```python
from build123d import *

# Parameters (mm, degrees)
F0_W     = 23.65
F0_H     = 51.55
F1_DEPTH = 35
F3_DEPTH = 23.651
F5_DEPTH = 6.25
F6_W     = 16.5
F6_H     = 4.038704
F7_DEPTH = 6.25


with BuildPart() as f1:
    # F0 (on Top) → F1 (new body)
    with BuildSketch(Plane.XY):
        with Locations((0.764201, -25.775)):
            Rectangle(F0_W, F0_H)
    extrude(amount=F1_DEPTH)

    # F2 (on face) → F3 (cut, through all)
    with BuildSketch(Plane.YZ.offset(12.589201)):
        Polygon((0, 28.75), (0, 35), (-15.663622, 35), (-11.5, 28.75), align=None)
    extrude(amount=-F3_DEPTH, mode=Mode.SUBTRACT)

    # F4 (on face) → F5 (cut)
    with BuildSketch(Plane.XY.offset(35)):
        Polygon((-4.985799, -47.763622), (0.764201, -47.763622), (6.514201, -47.763622), (9.014201, -43.008048), (9.014201, -15.663622), (0.764201, -15.663622), (-7.485799, -15.663622), (-7.485799, -43.008048), align=None)
    extrude(amount=-F5_DEPTH, mode=Mode.SUBTRACT)

    # F6 (on face) → F7 (cut)
    with BuildSketch(Plane.XY.offset(35)):
        with Locations((0.764201, -13.64427)):
            Rectangle(F6_W, F6_H)
    extrude(amount=-F7_DEPTH, mode=Mode.SUBTRACT)


solid = f1.part
```
Work out the finished part from the listing and answer in its coordinate system (mm). A direction names the side the tool comes from. Coordinates: 2 decimals unless noted, no trailing zeros. Loops run counter-clockwise (first coordinate to the right, second up) from the corner with the lowest first, then second, coordinate; pieces in that order, holes last. Notation, with made-up numbers: (70, -7) - (118, -7) arc R17 ccw to (118, 11) - close; hole circle Ø11 at (-16, 30). An arc over 180 degrees is marked (long way). Use a Markdown table: item, result.
Item 1: Given pin 1 Ø1.5 at (x, z) = (8.5, 31) entering from +Y; pin 2 Ø12.5 at (x, y) = (-0.5, -5) entering from +Z, each flat-ended and moving along its own axis, determine where each tip first touches the part or whether it passes through.
Evaluation:
| item | result |
|---|---|
| pin 1 | stops at y = -12.64 |
| pin 2 | stops at z = 28.75 |
Item 2: Find section B-B, the plane y = -21. Determine the outline of the cut face in (x, z), and give its area (3 significant figures).
Evaluation:
| item | result |
|---|---|
| outline | (-11.06, 0) - (12.59, 0) - (12.59, 35) - (9.01, 35) - (9.01, 28.75) - (-7.49, 28.75) - (-7.49, 35) - (-11.06, 35) - close |
| area | 725 mm2 |
Item 3: For faces 1 (the flat face through (1, -6, 28.75)), 2 (the flat face through (1, -29, 28.75)), 3 (the flat face through (-8, -38, 35)), determine the directions among +Z, -Z, +X, -X, +Y, -Y from which every point of the face is accessible in a straight line to the end or side of a thin tool.
Evaluation:
| item | result |
|---|---|
| face 1 | +Z, +X, -X, +Y |
| face 2 | +Z |
| face 3 | +Z, +X, -X, +Y, -Y |
Item 4: Find section C-C, the plane z = 29.5. Determine the outline of the cut face in (x, y), and give its area (3 significant figures).
Evaluation:
| item | result |
|---|---|
| outline | (-11.06, -51.55) - (12.59, -51.55) - (12.59, -12) - (9.01, -12) - (9.01, -43.01) - (6.51, -47.76) - (-4.99, -47.76) - (-7.49, -43.01) - (-7.49, -12) - (-11.06, -12) - close |
| area | 357 mm2 |
Item 5: Find section A-A, the plane x = -3.5. Determine the outline of the cut face in (y, z), and give its area (3 significant figures).
Evaluation:
| item | result |
|---|---|
| outline | (-51.55, 0) - (0, 0) - (0, 28.75) - (-11.5, 28.75) - (-11.62, 28.94) - (-11.62, 28.75) - (-47.76, 28.75) - (-47.76, 35) - (-51.55, 35) - close |
| area | 1,510 mm2 |
Item 6: Find section D-D, the plane y = -14.5. Determine the outline of the cut face in (x, z), and give its area (3 significant figures).
Evaluation:
| item | result |
|---|---|
| outline | (-11.06, 0) - (12.59, 0) - (12.59, 33.25) - (9.01, 33.25) - (9.01, 28.75) - (-7.49, 28.75) - (-7.49, 33.25) - (-11.06, 33.25) - close |
| area | 712 mm2 |
Item 7: Consider probe 1 along X at (y, z) = (-22.5, 32); probe 2 along Y at (x, z) = (1.25, 30.5); probe 3 along Z at (x, y) = (-8.75, -6.5). Determine where each line is inside the solid, lowest interval first. Write a range as from..to.
Evaluation:
| item | result |
|---|---|
| probe 1 | x = -11.06..-7.49, 9.01..12.59 |
| probe 2 | y = -51.55..-47.76 |
| probe 3 | z = 0..28.75 |
